The figure shows three views and two pictorial views of one solid part (mm, origin at its lowest corner). Answer the questions. A direction names the side the tool comes from. Give positions to 0.01 mm unless a question says otherwise; leave off trailing zeros. Loops run counter-clockwise (first coordinate to the right, second up) from the corner with the lowest first, then second, coordinate; pieces in that order, holes last. Notation, with made-up numbers: (69, 44) - (99, 44) arc R28 ccw to (99, 79) - close; hole circle Ø4 at (6, 36.25). An arc over 180 degrees is marked (long way). Use CSV: the item, a comma, the result in double quotes.
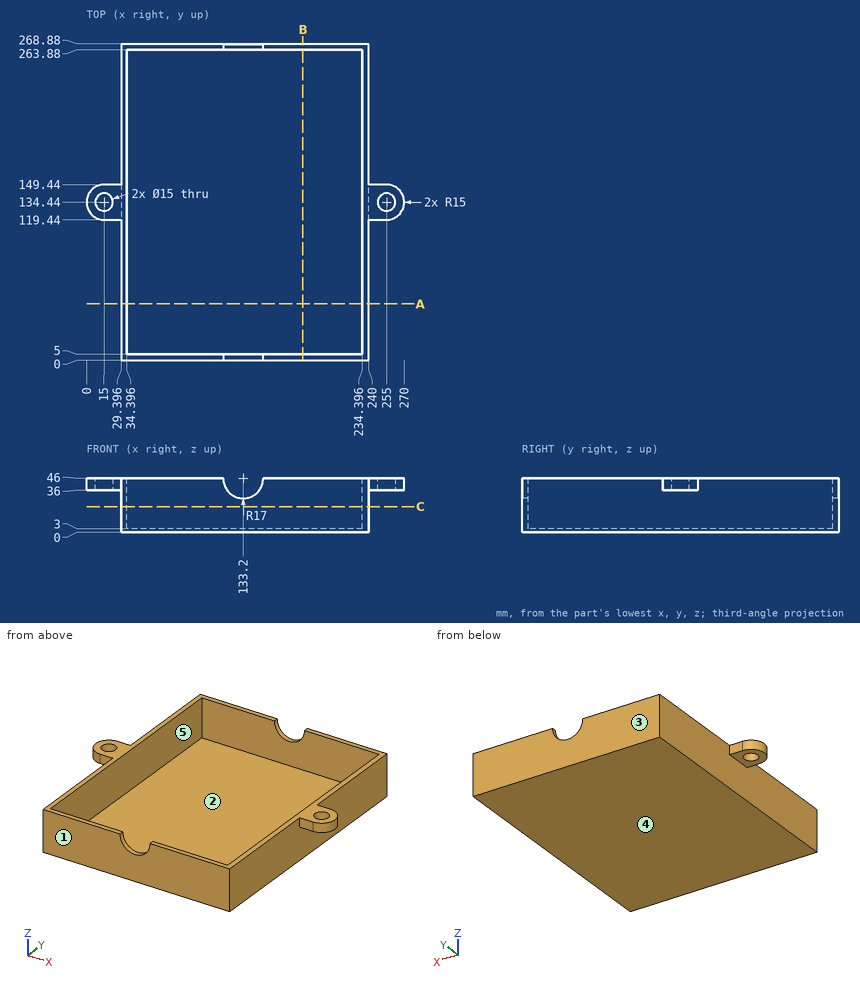
Item 1: Given P1, Ø14, axis at y = 132, z = 25.5, coming from the -X side; P2, Ø23.5, axis at x = 12.5, y = 139, coming from the -Z side; P3, Ø23, axis at y = 118.5, z = 22, coming from the +X side; P4, Ø9, axis at x = 255, y = 134.44, coming from the -Z side, each flat-ended and moving along its own axis, determine where each tip first touches the part or whether it passes through.
Determined:
P1,"stops at x = 29.4"
P2,"stops at z = 36"
P3,"stops at x = 240"
P4,"passes through"
Item 2: A cutting plane is placed at B-B on x = 184. Determine the outline of the cut face in (y, z), and give its area (3 significant figures).
Determined:
outline,"(0, 0) - (268.88, 0) - (268.88, 46) - (263.88, 46) - (263.88, 3) - (5, 3) - (5, 46) - (0, 46) - close"
area,"1,240 mm²"
Item 3: A cutting plane is placed at A-A on y = 48. Determine the outline of the cut face in (x, z), and give its area (3 significant figures).
Determined:
outline,"(29.4, 0) - (240, 0) - (240, 46) - (234.4, 46) - (234.4, 3) - (34.4, 3) - (34.4, 46) - (29.4, 46) - close"
area,"1,090 mm²"
Item 4: A cutting plane is placed at C-C on z = 22. Determine the outline of the cut face in (x, y).
Determined:
outline,"(29.4, 0) - (240, 0) - (240, 268.88) - (29.4, 268.88) - close; hole (34.4, 5) - (234.4, 5) - (234.4, 263.88) - (34.4, 263.88) - close"
Item 5: For the marked faces 1 and 2, determine the directions among +Z, -Z, +X, -X, +Y, -Y from which every point of the face is accessible in a straight line to the end or side of a thin tool.
Determined:
face 1,"+Z, -Z, +X, -X, -Y"
face 2,"+Z"
Item 6: The mould has two halves that part along Y. Classify the marked faces 3, 4 and 5: pulls with the +Y half, pulls with the -Y half, needs draft (parallel to the pull), parting line crosses it, or undercut.
Determined:
face 3,"pulls with the +Y half"
face 4,"needs draft"
face 5,"undercut"
Item 7: Find the intervals of material crossed by line 1 (X direction, y = 117.5, z = 25.5); line 2 (Y direction, x = 48.5, z = 19.5); line 3 (Z direction, x = 58, y = 192.5), in increasing order.
Determined:
line 1,"x = 29.4 to 34.4, 234.4 to 240"
line 2,"y = 0 to 5, 263.88 to 268.88"
line 3,"z = 0 to 3"
